Source: three-view drawing plus pictorial views. Frame: mm from the lowest corner of the part. A direction names the side the tool comes from. Coordinates: 2 decimals unless noted, no trailing zeros. Order: outer loops, then holes, each group sorted by start corner. A loop starts at its lowest first (then second) coordinate and runs counter-clockwise, first axis right, second up. Notation, with made-up numbers: M -39.75,-23 L -10.75,-23 A19 cw -10.75,-16 Z; hole C -32.5,56.5 d5. An arc over 180 degrees is marked long. Use CSV: the item, a comma, the result in double quotes. Start each with the question number.
Q1. Section query B-B, the plane y = 15.5. Output: boundary loops of the cut face in (x, z).
Q2. Ray query, probe 1 along X at (y, z) = (11, 1); probe 2 along Y at (x, z) = (0.75, 7); probe 3 along Z at (x, y) = (1.3, 10). Return the intervals inside material, ascending.
Q3. Section query C-C, the plane y = 10. Output: boundary loops of the cut face in (x, z).
Q4. Mould query, pull axis Y, two halves, no side actions, for the marked faces 3, 4, 5 and 6. Classes: +Y half, -Y half, draft (parallel to the pull), parting line (faces both ways), or undercut.
Q5. Section query A-A, the plane x = 7. Output: boundary loops of the cut face in (y, z), and give its area (3 significant figures).
Q6. First-contact query: P1, Ø3, axis at x = 6.5, y = 4, coming from the -Z side. Flat tip, straight axial feed; report the tip coordinate or a pass-through.
Q7. Access query for the marked faces 1 and 2. Directions: +Z, -Z, +X, -X, +Y, -Y. A direction counts if a zero-diameter tool reaches every point of the face in a straight line with its end or side. Return the directions, or none.
Q8. Section query D-D, the plane z = 11. Output: boundary loops of the cut face in (x, y).
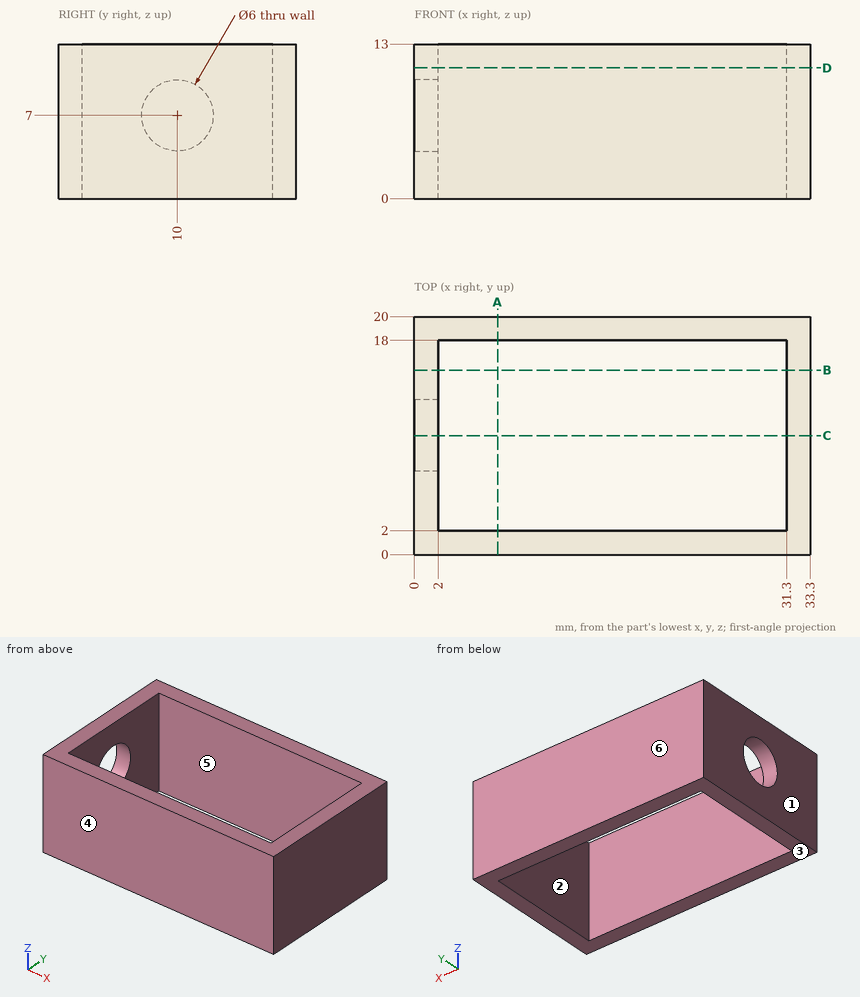
Responses:
1,outline,"M 0,0 L 2,0 L 2,13 L 0,13 Z; M 31.3,0 L 33.3,0 L 33.3,13 L 31.3,13 Z"
2,probe 1,"x = 0 to 2, 31.3 to 33.3"
2,probe 2,"y = 0 to 7, 13 to 20"
2,probe 3,"z = 0 to 4, 10 to 13"
3,outline,"M 0,0 L 2,0 L 2,4 L 0,4 Z; M 0,10 L 2,10 L 2,13 L 0,13 Z; M 31.3,0 L 33.3,0 L 33.3,13 L 31.3,13 Z"
4,face 3,"draft"
4,face 4,"-Y half"
4,face 5,"undercut"
4,face 6,"+Y half"
5,outline,"M 0,0 L 2,0 L 2,13 L 0,13 Z; M 18,0 L 20,0 L 20,13 L 18,13 Z"
5,area,"52.0 mm²"
6,P1,"passes through"
7,face 1,"+Z, -Z, -X, +Y, -Y"
7,face 2,"+Z, -Z"
8,outline,"M 0,0 L 33.3,0 L 33.3,20 L 0,20 Z; hole M 2,2 L 31.3,2 L 31.3,18 L 2,18 Z"
